from build123d import *

# Parameters (mm, degrees)
SKETCH1_W                                       = 317.5
SKETCH1_H                                       = 50.8
BOSS_EXTRUDE1_DEPTH                             = 6.35
CBORE_FOR_10_SOCKET_HEAD_CAP_SCREW1_D           = 5.1054
CBORE_FOR_10_SOCKET_HEAD_CAP_SCREW1_CBORE_D     = 9.525
CBORE_FOR_10_SOCKET_HEAD_CAP_SCREW1_CBORE_DEPTH = 4.826
F_1_4_CLEARANCE_HOLE2_D                         = 6.7564
F_6_32_TAPPED_HOLE1_D                           = 2.7051
SKETCH12_W                                      = 31.75
SKETCH12_H                                      = 25.4
BOSS_EXTRUDE3_DEPTH                             = 6.35
F_1_4_CLEARANCE_HOLE1_D                         = 6.7564
FILLET1_R                                       = 12.7
FILLET2_R                                       = 2.54


with BuildPart() as part:
    # Sketch1 → Boss-Extrude1 (new body)
    with BuildSketch(Plane(origin=(0, 0, 0), x_dir=(1, 0, 0), z_dir=(0, 1, 0))):
        Rectangle(SKETCH1_W, SKETCH1_H)
    extrude(amount=BOSS_EXTRUDE1_DEPTH)

    # CBORE for #10 Socket Head Cap Screw1 (through all)
    with Locations(Plane(origin=(0, 6.35, 0), x_dir=(1, 0, 0), z_dir=(0, 1, 0))):
        with Locations((-125.73, -12.7), (19.05, 12.7), (69.85, 12.7), (19.05, -12.7), (69.85, -12.7), (-125.73, 12.7), (-125.73, 0)):
            CounterBoreHole(CBORE_FOR_10_SOCKET_HEAD_CAP_SCREW1_D / 2, CBORE_FOR_10_SOCKET_HEAD_CAP_SCREW1_CBORE_D / 2, CBORE_FOR_10_SOCKET_HEAD_CAP_SCREW1_CBORE_DEPTH)

    # 1/4 Clearance Hole2 (through all)
    with Locations(Plane.XZ):
        with Locations((-146.05, 12.7), (-146.05, 0), (-146.05, -12.7), (146.05, 12.7), (146.05, 0), (146.05, -12.7)):
            Hole(F_1_4_CLEARANCE_HOLE2_D / 2)

    # #6-32 Tapped Hole1 (through all)
    with Locations(Plane(origin=(0, 0, 0), x_dir=(-1, 0, 0), z_dir=(0, -1, 0))):
        with Locations((57.15, 0)):
            Hole(F_6_32_TAPPED_HOLE1_D / 2)

    # Sketch12 → Boss-Extrude3 (add)
    with BuildSketch(Plane(origin=(0, 6.35, 0), x_dir=(1, 0, 0), z_dir=(0, 1, 0))):
        with Locations((-57.15, 38.1)):
            Rectangle(SKETCH12_W, SKETCH12_H)
    extrude(amount=-BOSS_EXTRUDE3_DEPTH)

    # 1/4 Clearance Hole1 (through all)
    with Locations(Plane(origin=(0, 0, 0), x_dir=(-1, 0, 0), z_dir=(0, -1, 0))):
        with Locations((62.23, 43.18), (52.07, 33.02)):
            Hole(F_1_4_CLEARANCE_HOLE1_D / 2)

    # Fillet1
    fillet1_edges = [part.edges().sort_by_distance(p)[0] for p in [
        (-73.025, 3.175, -25.4),
        (-41.275, 3.175, -25.4),
    ]]
    fillet(fillet1_edges, radius=FILLET1_R)

    # Fillet2
    fillet2_edges = [part.edges().sort_by_distance(p)[0] for p in [
        (158.75, 3.175, 25.4),
        (-158.75, 3.175, 25.4),
        (-158.75, 3.175, -25.4),
        (158.75, 3.175, -25.4),
    ]]
    fillet(fillet2_edges, radius=FILLET2_R)


solid = part.part
Model file for the job. Use its own axes, mm. A direction names the side the tool comes from. Give positions to 0.01 mm unless a question says otherwise; leave off trailing zeros. Order: outer loops, then holes, each group sorted by start corner. A loop starts at its lowest first (then second) coordinate and runs counter-clockwise, first axis right, second up. Notation, with made-up numbers: (13.5, -9) - (27.5, -9) arc R27 cw to (27.5, 23) - close; hole circle Ø9 at (34, 52.5). An arc over 180 degrees is marked (long way). Return JSON: item names as keys, results as strings.
1) Flat gauge pins, fed straight in: P1, Ø1.9, axis at x = 76.5, y = 3.5, coming from the -Z side; P2, Ø4, axis at x = 146.05, z = -12.7, coming from the +Y side; P3, Ø5.5, axis at x = 69.85, z = -12.7, coming from the +Y side. Where does each tip first touch, or does it go through?
Geometry says:
{"P1": "z = -25.4", "P2": "through", "P3": "y = 1.52"}
2) 3-axis set-ups, long thin cutter, end or side, ignore diameter. For faces 1 (the cylindrical face through (-142.675, 3.219, 0.149)), 2 (the flat face through (-73.025, 3, -44)), 3 (the flat face through (21, 1.524, 15)): which of +Z, -Z, +X, -X, +Y, -Y reach the whole face in a straight line?
Geometry says:
{"face 1": "+Y, -Y", "face 2": "-Z, -X, +Y, -Y", "face 3": "+Y"}
3) Cut at C-C, the plane z = -33.02. Give the cut face in (x, y), plus the area to 3 significant figures.
Geometry says:
{"outline": "(-74.09, 0) - (-55.45, 0) - (-55.45, 6.35) - (-74.09, 6.35) - close; (-48.69, 0) - (-40.21, 0) - (-40.21, 6.35) - (-48.69, 6.35) - close", "area": "172 mm²"}
4) Cut at B-B, the plane x = 146.05. Give the cut face in (y, z), plus the area to 3 significant figures.
Geometry says:
{"outline": "(0, -25.4) - (6.35, -25.4) - (6.35, -16.08) - (0, -16.08) - close; (0, -9.32) - (6.35, -9.32) - (6.35, -3.38) - (0, -3.38) - close; (0, 3.38) - (6.35, 3.38) - (6.35, 9.32) - (0, 9.32) - close; (0, 16.08) - (6.35, 16.08) - (6.35, 25.4) - (0, 25.4) - close", "area": "194 mm²"}
5) Cut at A-A, the plane x = -52.07. Give the cut face in (y, z), plus the area to 3 significant figures.
Geometry says:
{"outline": "(0, -50.8) - (6.35, -50.8) - (6.35, -36.4) - (0, -36.4) - close; (0, -29.64) - (6.35, -29.64) - (6.35, 25.4) - (0, 25.4) - close", "area": "441 mm²"}
6) Probe line 1 (Z direction, x = -125.73, y = 2.65); line 2 (Z direction, x = 146.05, y = 4.75); line 3 (Z direction, x = 69.85, y = 1). List the from-to ranges inside material, lowest first. Write a range as from..to.
Geometry says:
{"line 1": "-25.4..-17.46, -7.94..-4.76, 4.76..7.94, 17.46..25.4", "line 2": "-25.4..-16.08, -9.32..-3.38, 3.38..9.32, 16.08..25.4", "line 3": "-25.4..-15.25, -10.15..10.15, 15.25..25.4"}
7) Cut at D-D, the plane x = 102. Give the cut face in (y, z), plus the area to 3 significant figures.
Geometry says:
{"outline": "(0, -25.4) - (6.35, -25.4) - (6.35, 25.4) - (0, 25.4) - close", "area": "323 mm²"}
8) Pull direction Z, two halves, no side cores. Call faces 4 (the cylindrical face through (-37.456, 3.131, -29.022)), 5 (the flat face through (72, 1.524, -11)), 6 (the flat face through (-158.75, 3, 0)): pulls with the +Z half, pulls with the -Z half, needs draft (parallel to the pull), parting line crosses it, or undercut.
Geometry says:
{"face 4": "pulls with the -Z half", "face 5": "undercut", "face 6": "needs draft"}
